Here's how the part is built. I have some questions about the finished solid (model axes, mm). A direction names the side the tool comes from. Coordinates: 2 decimals unless noted, no trailing zeros. Loops run counter-clockwise (first coordinate to the right, second up) from the corner with the lowest first, then second, coordinate; pieces in that order, holes last. Notation, with made-up numbers: M 36,-34.5 L 72,-34.5 A22 ccw 72,-28.5 Z; hole C 89,31 d2. An arc over 180 degrees is marked long. Use CSV: the item, a comma, the result in double quotes. Start each with the question number.
Q1. If we mould it in two halves opening along Y, with no side actions, what happens to faces 4 (the flat face through (6, -147, -146.598)), 5 (the cylindrical face through (6.26, 53.5, -15.59)), 6 (the cylindrical face through (6.261, 30.935, -26.36))? For each: +Y half, -Y half, draft (parallel to the pull), parting line (faces both ways), or undercut.
Q2. If we section it at A-A (x = 9.5): Please give me the cut outline in (y, z) (3 decimals).
Q3. If we section it at C-C (y = -122): Please give me the cut outline in (x, z), and give its area (3 significant figures).
Q4. Which directions (+Z, -Z, +X, -X, +Y, -Y) give clear straight access to the entire face, cutting with the end or side of a thin tool? Please do faces 1 (the flat face through (6, 58.73, -45)), 2 (the cylindrical face through (6.26, -129.98, -56.71)), 3 (the flat face through (6, 46, -51.598)).
Q5. Please list where these lines run through material, in increasing order: probe 1 along Y at (x, z) = (5.25, -104); probe 2 along Z at (x, y) = (6.75, 6.5); probe 3 along Z at (x, y) = (2, -125). Write a range as [from, to].
Q6. For pin 1 Ø4 at (x, z) = (5, -48) entering from -Y; pin 2 Ø6.5 at (x, z) = (5.5, -103) entering from +Y; pin 3 Ø5 at (x, y) = (6.5, -86.5) entering from -Z, each with a flat end and sliding along its axis, tell me the tip position at first contact or that it passes through.
Q7. If we section it at B-B (z = -135): Please give me the cut outline in (x, y), and give its area (4 significant figures).
from build123d import *

# Parameters (mm, degrees)
F1_DEPTH = 12.7


with BuildPart() as f1:
    # F0 (on Right) → F1 (new body)
    with BuildSketch(Plane.YZ):
        with BuildLine():
            ThreePointArc((-127.4130486986, -23.8944376975), (-150.5555928046, -42.505234855), (-159.2704062288, -70.8952180447))
            Line((-159.2704062288, -70.8952180447), (-159.2704062288, -146.5982919273))
            Line((-159.2704062288, -146.5982919273), (-134.2704062288, -146.5982919273))
            Line((-134.2704062288, -146.5982919273), (-134.2704062288, -70.8952180447))
            Line((-134.2704062288, -70.8952180447), (-134.2704062288, -53.5434135268))
            Line((-134.2704062288, -53.5434135268), (-118.1528498499, -47.1161671181))
            Line((-118.1528498499, -47.1161671181), (-13.3015476427, -5.3042981397))
            Line((-13.3015476427, -5.3042981397), (0, 0))
            Line((0, 0), (11.4811224988, -8.5586549536))
            Line((11.4811224988, -8.5586549536), (23.4298202916, -17.4658660356))
            Line((23.4298202916, -17.4658660356), (33.7295937712, -25.143878993))
            Line((33.7295937712, -25.143878993), (33.7295937712, -37.9905601483))
            Line((33.7295937712, -37.9905601483), (33.7295937712, -51.5982919273))
            Line((33.7295937712, -51.5982919273), (58.7295937712, -51.5982919273))
            Line((58.7295937712, -51.5982919273), (58.7295937712, -37.9905601483))
            ThreePointArc((58.7295937712, -37.9905601483), (53.3545747633, -15.295602685), (38.371447753, 2.577780559))
            Line((38.371447753, 2.577780559), (26.4227499601, 11.4849916409))
            ThreePointArc((26.4227499601, 11.4849916409), (2.7689181611, 21.0859439695), (-22.5617464914, 17.9174312808))
            Line((-22.5617464914, 17.9174312808), (-127.4130486986, -23.8944376975))
        make_face()
        with BuildLine():
            Line((-134.2704062288, -53.5434135268), (-134.2704062288, -70.8952180447))
            ThreePointArc((-134.2704062288, -70.8952180447), (-129.8613306624, -56.5319063914), (-118.1528498499, -47.1161671181))
            Line((-118.1528498499, -47.1161671181), (-134.2704062288, -53.5434135268))
        make_face()
        with BuildLine():
            Line((0, 0), (-13.3015476427, -5.3042981397))
            ThreePointArc((-13.3015476427, -5.3042981397), (-0.4860335102, -3.7012561471), (11.4811224988, -8.5586549536))
            Line((11.4811224988, -8.5586549536), (0, 0))
        make_face()
        with BuildLine():
            Line((33.7295937712, -25.143878993), (23.4298202916, -17.4658660356))
            ThreePointArc((23.4298202916, -17.4658660356), (31.0102165656, -26.5085263329), (33.7295937712, -37.9905601483))
            Line((33.7295937712, -37.9905601483), (33.7295937712, -25.143878993))
        make_face()
    extrude(amount=F1_DEPTH)


solid = f1.part
Results below:
1,face 4,"draft"
1,face 5,"+Y half"
1,face 6,"undercut"
2,outline,"M -159.27,-146.598 L -134.27,-146.598 L -134.27,-70.895 A25.6 cw -118.153,-47.116 L -13.302,-5.304 A25.6 cw 11.481,-8.559 L 23.43,-17.466 A25.6 cw 33.73,-37.991 L 33.73,-51.598 L 58.73,-51.598 L 58.73,-37.991 A50.6 ccw 38.371,2.578 L 26.423,11.485 A50.6 ccw -22.562,17.917 L -127.413,-23.894 A50.6 ccw -159.27,-70.895 Z"
3,outline,"M 0,-49.04 L 12.7,-49.04 L 12.7,-21.74 L 0,-21.74 Z"
3,area,"347 mm^2"
4,face 1,"+Z, -Z, +X, -X, +Y"
4,face 2,"-Z, +X, -X"
4,face 3,"-Z, +X, -X, +Y"
5,probe 1,"[-159.27, -134.27]"
5,probe 2,"[-5.66, 20.45]"
5,probe 3,"[-51.18, -22.93]"
6,pin 1,"y = -154.75"
6,pin 2,"y = -134.27"
6,pin 3,"z = -35.49"
7,outline,"M 0,-159.27 L 12.7,-159.27 L 12.7,-134.27 L 0,-134.27 Z"
7,area,"317.5 mm^2"
